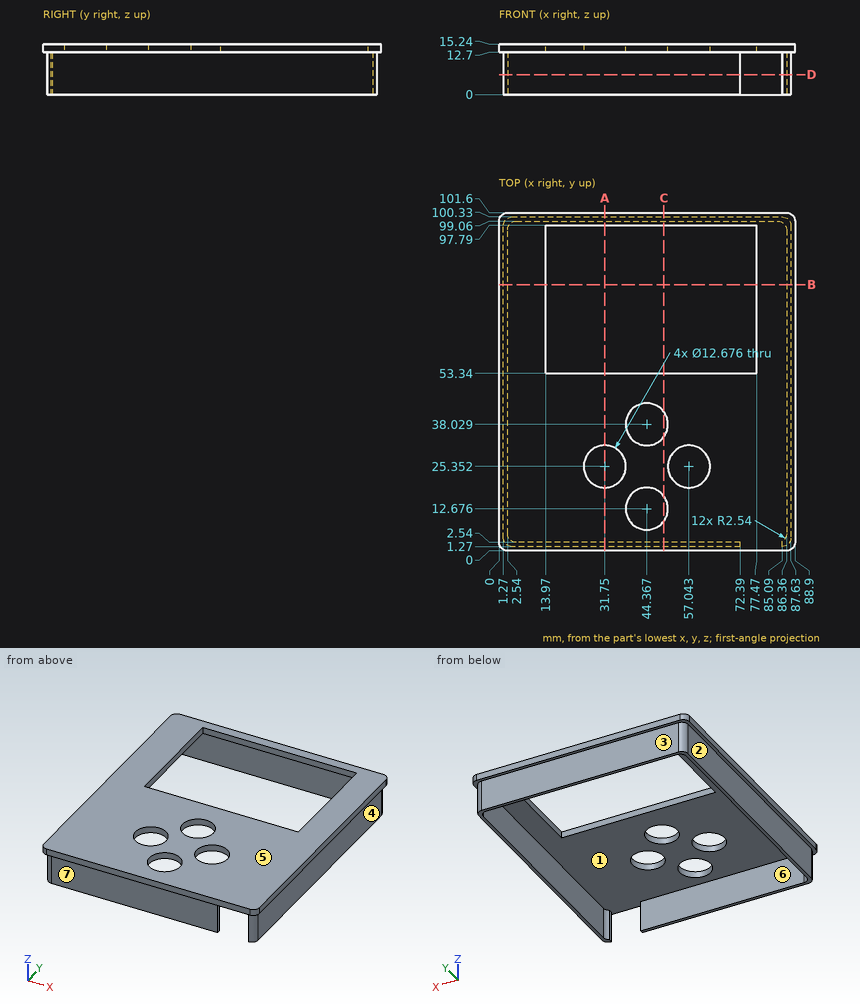
The figure shows three views and two pictorial views of one solid part (mm, origin at its lowest corner). Answer the questions. A direction names the side the tool comes from. Coordinates: 2 decimals unless noted, no trailing zeros. Loops run counter-clockwise (first coordinate to the right, second up) from the corner with the lowest first, then second, coordinate; pieces in that order, holes last. Notation, with made-up numbers: (38, 32.5) -> (80, 32.5) arc R22 ccw to (80, 47.5) -> close; hole circle Ø1 at (-6.5, 21). An arc over 180 degrees is marked (long way). Write item = value, one per line. Start each with the question number.
1) A cutting plane is placed at B-B (y = 80). Give the vertices of the cut face in (x, z).
2) Straight lines are drawn through the part: line 1 (Y direction, x = 31.75, z = 13.8) (1 decimal); line 2 (X direction, y = 28, z = 7.5); line 3 (Y direction, x = 57, z = 10.5). For each, find the intervals that lie inside material, in ascending order. Write a range as from..to.
3) A cutting plane is placed at C-C (x = 49.5). Give the vertices of the cut face in (y, z) (1 decimal).
4) A cutting plane is placed at D-D (z = 6). Give the vertices of the cut face in (x, y).
5) Given pin 1 Ø1 at (x, z) = (54.5, 11.5) entering from +Y; pin 2 Ø4 at (x, y) = (35.5, 43.5) entering from -Z; pin 3 Ø1 at (y, z) = (2, 8) entering from +X (1 decimal); pin 4 Ø16.5 at (x, y) = (31.75, 25.35) entering from +Z, each flat-ended and moving along its own axis, determine where each tip first touches the part or whether it passes through.
6) A tool of negligible diameter and unlimited length cuts with its end or side. For the marked faces 5, 6 and 7, from which of +Z, -Z, +X, -X, +Y, -Y can it reach the whole face along a straight path? Write none if from no direction.
7) A cutting plane is placed at A-A (x = 31.75). Give the vertices of the cut face in (y, z) (1 decimal), then the cut area to 3 significant figures.
8) The mould has two halves that part along X. Classify the marked faces 1, 2, 3 and 4: released by +X, released by -X, zero draft, split by the parting line, or undercut.
Responses:
q1.outline = (0, 12.7) -> (1.27, 12.7) -> (1.27, 0) -> (2.54, 0) -> (2.54, 12.7) -> (13.97, 12.7) -> (13.97, 15.24) -> (0, 15.24) -> close; (77.47, 12.7) -> (86.36, 12.7) -> (86.36, 0) -> (87.63, 0) -> (87.63, 12.7) -> (88.9, 12.7) -> (88.9, 15.24) -> (77.47, 15.24) -> close
q2.line_1 = 0..19, 31.7..53.3, 97.8..101.6
q2.line_2 = 1.27..2.54, 86.36..87.63
q2.line_3 = 1.27..2.54, 99.06..100.33
q3.outline = (0, 12.7) -> (1.3, 12.7) -> (1.3, 0) -> (2.5, 0) -> (2.5, 12.7) -> (9, 12.7) -> (9, 15.2) -> (0, 15.2) -> close; (16.4, 12.7) -> (34.3, 12.7) -> (34.3, 15.2) -> (16.4, 15.2) -> close; (41.7, 12.7) -> (53.3, 12.7) -> (53.3, 15.2) -> (41.7, 15.2) -> close; (97.8, 12.7) -> (99.1, 12.7) -> (99.1, 0) -> (100.3, 0) -> (100.3, 12.7) -> (101.6, 12.7) -> (101.6, 15.2) -> (97.8, 15.2) -> close
q4.outline = (1.27, 3.81) arc R2.54 ccw to (3.81, 1.27) -> (72.39, 1.27) -> (72.39, 2.54) -> (5.08, 2.54) arc R2.54 cw to (2.54, 5.08) -> (2.54, 96.52) arc R2.54 cw to (5.08, 99.06) -> (83.82, 99.06) arc R2.54 cw to (86.36, 96.52) -> (86.36, 5.08) arc R2.54 cw to (85.09, 2.88) -> (85.09, 1.27) arc R2.54 ccw to (87.63, 3.81) -> (87.63, 97.79) arc R2.54 ccw to (85.09, 100.33) -> (3.81, 100.33) arc R2.54 ccw to (1.27, 97.79) -> close
q5.pin_1 = 100.33
q5.pin_2 = 12.7
q5.pin_3 = 87.3
q5.pin_4 = 15.24
q6.face_5 = +Z, +X, -X, +Y, -Y
q6.face_6 = -Z
q6.face_7 = -Z, +X, -X, -Y
q7.outline = (0, 12.7) -> (1.3, 12.7) -> (1.3, 0) -> (2.5, 0) -> (2.5, 12.7) -> (19, 12.7) -> (19, 15.2) -> (0, 15.2) -> close; (31.7, 12.7) -> (53.3, 12.7) -> (53.3, 15.2) -> (31.7, 15.2) -> close; (97.8, 12.7) -> (99.1, 12.7) -> (99.1, 0) -> (100.3, 0) -> (100.3, 12.7) -> (101.6, 12.7) -> (101.6, 15.2) -> (97.8, 15.2) -> close
q7.area = 145 mm²
q8.face_1 = undercut
q8.face_2 = released by -X
q8.face_3 = zero draft
q8.face_4 = released by +X
